from build123d import *

# Parameters (mm, degrees)
SKETCH_1_R               = 2
EXTRUDE_1_DEPTH          = 60
SKETCH_3_W               = 4.2
SKETCH_3_H               = 1
CUT_EXTRUDE_1_DEPTH      = 8
CUT_EXTRUDE_2_REACH      = 62.128
SKETCH_4_W               = 1
SKETCH_4_H               = 4
SKETCH_6_W               = 4.2
SKETCH_6_H               = 1
CUT_EXTRUDE_3_DEPTH      = 8
CUT_EXTRUDE_4_DEPTH      = 61.073621499
CUT_EXTRUDE_4_DEPTH_BACK = 61.073621499
SKETCH_7_W               = 1
SKETCH_7_H               = 4


with BuildPart() as part:
    # 草图1 → 凸台-拉伸1 (new body)
    with BuildSketch(Plane.XY):
        Circle(SKETCH_1_R)
    extrude(amount=-EXTRUDE_1_DEPTH)

    # 草图2 → 旋转1 (revolve)
    with BuildSketch(Plane(origin=(0, 0, 0), x_dir=(1, 0, 0), z_dir=(0, 1, 0))):
        Polygon((0, 0), (0, 2), (2.2, 2), (2, 0), align=None)
    revolve(axis=Axis((0, 0, 0), (0, 0, -1)))

    # 草图3 → 切除-拉伸1 (cut)
    with BuildSketch(Plane.XY):
        with Locations((0, 1.75)):
            Rectangle(SKETCH_3_W, SKETCH_3_H)
        with Locations((0, -1.75)):
            Rectangle(SKETCH_3_W, SKETCH_3_H)
    extrude(amount=-CUT_EXTRUDE_1_DEPTH, mode=Mode.SUBTRACT)

    # 草图4 → 切除-拉伸2 (cut, up to next)
    with BuildSketch(Plane.XZ.offset(1.25), mode=Mode.PRIVATE) as cut_extrude_2_sk1:
        with Locations((0, -2)):
            Rectangle(SKETCH_4_W, SKETCH_4_H)
    cut_extrude_2_tool1 = extrude(cut_extrude_2_sk1.sketch, amount=-CUT_EXTRUDE_2_REACH, mode=Mode.PRIVATE) & part.part
    add(cut_extrude_2_tool1.solids().sort_by_distance((0, -1.25, -2))[0], mode=Mode.SUBTRACT)

    # 草图5 → 旋转2 (revolve)
    with BuildSketch(Plane(origin=(0, 0, 0), x_dir=(1, 0, 0), z_dir=(0, 1, 0))):
        Polygon((0, 60), (0, 58), (2.2, 58), (2, 60), align=None)
    revolve(axis=Axis((0, 0, -58.137689197), (0, 0, -1)))

    # 草图6 → 切除-拉伸3 (cut)
    with BuildSketch(Plane(origin=(0, 0, -60), x_dir=(-1, 0, 0), z_dir=(0, 0, -1))):
        with Locations((0, 1.75)):
            Rectangle(SKETCH_6_W, SKETCH_6_H)
        with Locations((0, -1.75)):
            Rectangle(SKETCH_6_W, SKETCH_6_H)
    extrude(amount=-CUT_EXTRUDE_3_DEPTH, mode=Mode.SUBTRACT)

    # 草图7 → 切除-拉伸4 (cut, two sides: drawn at the far end of the back side and taken through both)
    with BuildSketch(Plane(origin=(0, 0, 0), x_dir=(1, 0, 0), z_dir=(0, 1, 0)).offset(-CUT_EXTRUDE_4_DEPTH_BACK)):
        with Locations((0, 58)):
            Rectangle(SKETCH_7_W, SKETCH_7_H)
    extrude(amount=CUT_EXTRUDE_4_DEPTH + CUT_EXTRUDE_4_DEPTH_BACK, mode=Mode.SUBTRACT)


solid = part.part
Geometry check sheet. Reference: the model listing, model coordinates, mm. A direction names the side the tool comes from. Coordinates: 2 decimals unless noted, no trailing zeros. Loops run counter-clockwise (first coordinate to the right, second up) from the corner with the lowest first, then second, coordinate; pieces in that order, holes last. Notation, with made-up numbers: (16.25, -29) - (35.25, -29) arc R14 ccw to (35.25, -22) - close; hole circle Ø3 at (52, 49). An arc over 180 degrees is marked (long way). Use one line per item in the form item = value. Start each with the question number.
Item 1: Section check B-B, the plane y = 0. Enter the section's corners in (x, z), and give its area (3 significant figures).
Item 2: Section check C-C, the plane z = -12.5. Enter the section's corners in (x, y).
Item 3: Section check A-A, the plane x = 0. Enter the section's corners in (y, z).
Item 4: Gauge pin test, flat ends, axial feed: pin 1 (0.8 mm diameter, centred on y = -0.5, z = -1.5, fed in from -X); pin 2 (1.8 mm diameter, centred on x = -0.5, z = -5.5, fed in from -Y); pin 3 (0.6 mm diameter, centred on x = 0, y = 1.5, fed in from +Z). Record the tip position at first contact, or that the pin passes through.
Item 5: Mould release check, pull along X, two halves, no side actions. Record for faces 1 (the face through (0, 1.25, -55)), 2 (the face through (0, 0, -4)), 3 (the face through (2.1, 0, -1)), 4 (the face through (-0.5, 0, -2)): +X half, -X half, draft (parallel to the pull), parting line (faces both ways), or undercut.
Item 6: Thickness scan on probe 1 along Y at (x, z) = (-1.25, -48.5); probe 2 along Y at (x, z) = (0.1, -47); probe 3 along X at (y, z) = (0.85, -2.5). Record the ranges inside material, lowest first.
Item 7: Tool access check on faces 5 (the face through (0, 1.25, -5)), 6 (the face through (0, -1.25, -55)), 7 (the face through (0, -2, -30)), 8 (the face through (0.5, 0, -58)), 9 (the face through (0.5, 0, -2)). Record the directions out of +Z, -Z, +X, -X, +Y, -Y that give a thin tool (end or side, any length) a straight path to the whole face; none if there is none.
Computed:
q1.outline = (-2.2, -58) - (-2, -60) - (-0.5, -60) - (-0.5, -56) - (0.5, -56) - (0.5, -60) - (2, -60) - (2.2, -58) - (2, -58) - (2, -2) - (2.2, -2) - (2, 0) - (0.5, 0) - (0.5, -4) - (-0.5, -4) - (-0.5, 0) - (-2, 0) - (-2.2, -2) - (-2, -2) - (-2, -58) - close
q1.area = 233 mm2
q2.outline = circle Ø4 at (0, 0)
q3.outline = (-2, -52) - (-1.25, -52) - (-1.25, -56) - (1.25, -56) - (1.25, -52) - (2, -52) - (2, -8) - (1.25, -8) - (1.25, -4) - (-1.25, -4) - (-1.25, -8) - (-2, -8) - close
q4.pin_1 = -2.17
q4.pin_2 = -1.25
q4.pin_3 = -4
q5.face_1 = draft
q5.face_2 = undercut
q5.face_3 = +X half
q5.face_4 = undercut
q6.probe_1 = -1.56 to 1.56
q6.probe_2 = -2 to 2
q6.probe_3 = -1.81 to -0.5, 0.5 to 1.81
q7.face_5 = +Z, +X, -X, +Y
q7.face_6 = -Z, +X, -X, -Y
q7.face_7 = none
q7.face_8 = -Z, +Y, -Y
q7.face_9 = +Z, +Y, -Y
